Autodesk Inventor part; units mm, degrees
ref_plane "YZ Plane" through (0, 0, 0) normal (1, 0, 0) x (0, 1, 0)
ref_plane "XZ Plane" through (0, 0, 0) normal (0, 1, 0) x (-1, 0, 0)
ref_plane "XY Plane" through (0, 0, 0) normal (0, 0, 1) x (1, 0, 0)
sketch "Sketch1" plane through (0, 0, 0) normal (0, 0, 1) x (1, 0, 0)
  circle A0 centre (0, 0) radius 20.8915
  circle A1 centre (0, 0) radius 15.24
  line L0 (-9.2613, 12.1031) -> (9.2613, 12.1031)
  line L1 (-9.2613, -12.1031) -> (9.2613, -12.1031)
  circle A2 centre (0, 0) radius 18.4404
  dimension "d0" = 41.783
  dimension "d1" = 30.48
  dimension "d2" = 12.1031
  dimension "d3" = 12.1031
  dimension "d4" = 36.8808
extrude "Extrusion1" add sketch "Sketch1" against normal blind 9.2964 contours A0
extrude "Extrusion2" add sketch "Sketch1" along normal blind 2.032 contours A0 | L0 A1 | A1 L1 | A2
thread "Thread1"
properties part number "Spring torque cap"
The model under review builds one solid part; all positions refer to its coordinate system, in mm. A direction names the side the tool comes from. Give positions to 0.01 mm unless a question says otherwise; leave off trailing zeros. Write each loop counter-clockwise with the first axis right and the second up, starting at its lowest first coordinate (ties: lowest second). Pieces come first, ordered by that corner, then holes. Notation, with made-up numbers: (-11.75, 52) -> (31.25, 52) arc R22 ccw to (31.25, 60) -> close; hole circle Ø9 at (77, -27.5). An arc over 180 degrees is marked (long way). Put each result on its own line as item: value.
(1) For pin 1 Ø2 at (y, z) = (-3.5, -7) entering from -X; pin 2 Ø0.6 at (x, z) = (-3, 1) entering from -Y; pin 3 Ø1.6 at (x, z) = (-1.5, 1) entering from +Y; pin 4 Ø22 at (x, y) = (0, 0) entering from +Z, all flat-tipped, find the tip position at first contact; note any pin that passes through.
Results are:
pin 1: x = -20.74
pin 2: y = -20.72
pin 3: y = 20.88
pin 4: through
(2) We need section A-A, the plane y = 0. Give the boundary of the cut face in (x, z), and give its area (3 significant figures).
Results are:
outline: (-20.89, -9.3) -> (-18.44, -9.3) -> (-18.44, 0) -> (-15.24, 0) -> (-15.24, 2.03) -> (-20.89, 2.03) -> close; (15.24, 0) -> (18.44, 0) -> (18.44, -9.3) -> (20.89, -9.3) -> (20.89, 2.03) -> (15.24, 2.03) -> close
area: 68.5 mm²
(3) To check wall thickness, follow probe 1 along Y at (x, z) = (0, -4); probe 2 along Y at (x, z) = (10, -2.5); probe 3 along X at (y, z) = (4.5, -2). State the ranges of each line that lie inside material, in increasing order. Write a range as from..to.
Results are:
probe 1: -20.89..-18.44, 18.44..20.89
probe 2: -18.34..-15.49, 15.49..18.34
probe 3: -20.4..-17.88, 17.88..20.4
(4) The part is to be moulded in two halves that separate along Y. For faces 1 (the flat face through (8, -17, -9.296)), 2 (the cylindrical face through (19.927, 6.275, -3.553)), 3 (the flat face through (0, -12.103, 1)), say which applies: pulls with the +Y half, pulls with the -Y half, needs draft (parallel to the pull), parting line crosses it, or undercut.
Results are:
face 1: needs draft
face 2: parting line crosses it
face 3: undercut
(5) Tool access review of faces 4 (the flat face through (0, -14, 2.032)), 5 (the flat face through (-0.1, 12.4, 0)), 6 (the cylindrical face through (-15.24, -0.2, 1)): name each direction out of +Z, -Z, +X, -X, +Y, -Y from which nothing blocks a thin tool from reaching the whole face with its end or side.
Results are:
face 4: +Z, +X, -X, +Y, -Y
face 5: -Z
face 6: +Z, -Z
(6) We need section C-C, the plane z = -7.5. Give the boundary of the cut face in (x, y), and give its area (3 significant figures).
Results are:
outline: circle Ø41.78 at (0, 0); hole circle Ø36.88 at (0, 0)
area: 303 mm²
(7) We need section B-B, the plane x = 0. Give the boundary of the cut face in (y, z), and give its area (3 significant figures).
Results are:
outline: (-20.89, -9.3) -> (-18.44, -9.3) -> (-18.44, 0) -> (-12.1, 0) -> (-12.1, 2.03) -> (-20.89, 2.03) -> close; (12.1, 0) -> (18.44, 0) -> (18.44, -9.3) -> (20.89, -9.3) -> (20.89, 2.03) -> (12.1, 2.03) -> close
area: 81.3 mm²
